The listing builds one solid part. Answer for the finished solid, in the listing's coordinates (mm). Coordinates: 2 decimals unless noted, no trailing zeros. Loops run counter-clockwise (first coordinate to the right, second up) from the corner with the lowest first, then second, coordinate; pieces in that order, holes last. Notation, with made-up numbers: M -2,35 L 25,35 A23 cw 25,47 Z; hole C 22.25,29 d9. An arc over 180 degrees is marked long. Return JSON: item names as keys, results as strings. Group by question number.
1. Section B-B (x = -1688) is taken. Write down the section's boundary in (y, z), then the cut area to 3 significant figures.
2. Section A-A (y = 458.5) is taken. Write down the section's boundary in (x, z), then the cut area to 3 significant figures.
3. Given P1, Ø12, axis at x = -1340.5, y = 682.5, coming from the -Z side, flat-ended and moving along its own axis, determine where the tip first touches the part or whether it passes through.
4. Section C-C (z = 5.75) is taken. Count the separate pieces of the cut face and the enclosed holes in it, then the cut area to 3 significant figures.
5. Straight lines are drawn through the part: L1, parallel to Y at x = -1674.5, z = 6.25; L2, parallel to X at y = 683.5, z = 4; L3, parallel to X at y = 1047, z = 6.25. For each, find the intervals that lie inside material, in ascending order. Write a range as from..to.
```python
from build123d import *

# Parameters (mm, degrees)
SKETCH1_W           = 18
SKETCH1_H           = 100
SKETCH1_W_2         = 100
SKETCH1_H_2         = 18
BOSS_EXTRUDE2_DEPTH = 18


with BuildPart() as part:
    # Sketch1 → Boss-Extrude2 (new body)
    with BuildSketch(Plane.XY):
        with BuildLine():
            Line((-1197.056949538, 402.692318001), (-1817.056949538, 402.692318001))
            Line((-1817.056949538, 402.692318001), (-1817.056949538, 1102.692318001))
            Line((-1817.056949538, 1102.692318001), (-1297.056949538, 1102.692318001))
            ThreePointArc((-1297.056949538, 1102.692318001), (-1226.346271419, 1073.402996119), (-1197.056949538, 1002.692318001))
            Line((-1197.056949538, 1002.692318001), (-1197.056949538, 402.692318001))
        make_face()
        with Locations((-1802.056949538, 1022.692318001)):
            Rectangle(SKETCH1_W, SKETCH1_H, mode=Mode.SUBTRACT)
        with Locations((-1802.056949538, 482.692318001)):
            Rectangle(SKETCH1_W, SKETCH1_H, mode=Mode.SUBTRACT)
        with Locations((-1352.056949538, 417.692318001)):
            Rectangle(SKETCH1_W_2, SKETCH1_H_2, mode=Mode.SUBTRACT)
        with Locations((-1662.056949538, 417.692318001)):
            Rectangle(SKETCH1_W_2, SKETCH1_H_2, mode=Mode.SUBTRACT)
        with Locations((-1662.056949538, 549.692318001)):
            Rectangle(SKETCH1_W_2, SKETCH1_H_2, mode=Mode.SUBTRACT)
        with Locations((-1352.056949538, 549.692318001)):
            Rectangle(SKETCH1_W_2, SKETCH1_H_2, mode=Mode.SUBTRACT)
        with Locations((-1662.056949538, 681.692318001)):
            Rectangle(SKETCH1_W_2, SKETCH1_H_2, mode=Mode.SUBTRACT)
        with Locations((-1352.056949538, 681.692318001)):
            Rectangle(SKETCH1_W_2, SKETCH1_H_2, mode=Mode.SUBTRACT)
        with Locations((-1662.056949538, 813.692318001)):
            Rectangle(SKETCH1_W_2, SKETCH1_H_2, mode=Mode.SUBTRACT)
        with Locations((-1352.056949538, 813.692318001)):
            Rectangle(SKETCH1_W_2, SKETCH1_H_2, mode=Mode.SUBTRACT)
    extrude(amount=BOSS_EXTRUDE2_DEPTH)


solid = part.part
```
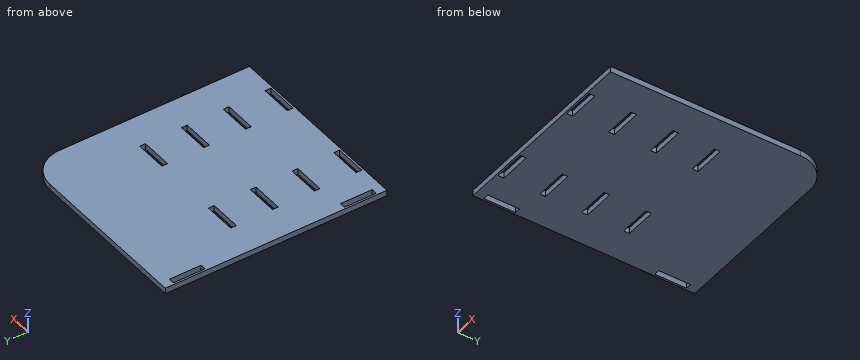
Worked out:
{
 "1": {"outline": "M 402.69,0 L 408.69,0 L 408.69,18 L 402.69,18 Z; M 426.69,0 L 540.69,0 L 540.69,18 L 426.69,18 Z; M 558.69,0 L 672.69,0 L 672.69,18 L 558.69,18 Z; M 690.69,0 L 804.69,0 L 804.69,18 L 690.69,18 Z; M 822.69,0 L 1102.69,0 L 1102.69,18 L 822.69,18 Z", "area": "11,300 mm^2"},
 "2": {"outline": "M -1817.06,0 L -1811.06,0 L -1811.06,18 L -1817.06,18 Z; M -1793.06,0 L -1197.06,0 L -1197.06,18 L -1793.06,18 Z", "area": "10,800 mm^2"},
 "3": {"P1": "through"},
 "4": {"separate pieces": "1", "enclosed holes": "10", "area": "414,000 mm^2"},
 "5": {"L1": "402.69..408.69, 426.69..540.69, 558.69..672.69, 690.69..804.69, 822.69..1102.69", "L2": "-1817.06..-1712.06, -1612.06..-1402.06, -1302.06..-1197.06", "L3": "-1817.06..-1811.06, -1793.06..-1207.41"}
}
